from build123d import *

# Parameters (mm, degrees)
ESBO_O1_W                = 125
ESBO_O1_H                = 175
RESSALTO_EXTRUS_O1_DEPTH = 5
ESBO_O2_W                = 2.5
ESBO_O2_H                = 49
RESSALTO_EXTRUS_O2_DEPTH = 5.4
FILETE1_R                = 2
ESBO_O3_R                = 1.35
CORTE_EXTRUS_O2_DEPTH    = 140.879984272
CORTE_EXTRUS_O3_DEPTH    = 108.664571703


with BuildPart() as part:
    # Esboço1 → Ressalto-extrusão1 (new body)
    with BuildSketch(Plane.XY):
        Rectangle(ESBO_O1_W, ESBO_O1_H)
    extrude(amount=RESSALTO_EXTRUS_O1_DEPTH)

    # Esboço2 → Ressalto-extrusão2 (add)
    with BuildSketch(Plane(origin=(0, 0, 0), x_dir=(-1, 0, 0), z_dir=(0, 0, -1))):
        with Locations((7.75, 0)):
            Rectangle(ESBO_O2_W, ESBO_O2_H)
        with Locations((45.25, 0)):
            Rectangle(ESBO_O2_W, ESBO_O2_H)
    extrude(amount=RESSALTO_EXTRUS_O2_DEPTH)

    # Filete1
    filete1_edges = [part.edges().sort_by_distance(p)[0] for p in [
        (-7.75, 24.5, -5.4),
        (-7.75, -24.5, -5.4),
        (-45.25, 24.5, -5.4),
        (-45.25, -24.5, -5.4),
    ]]
    fillet(filete1_edges, radius=FILETE1_R)

    # Esboço3 → Corte-extrusão2 (cut, through all)
    with BuildSketch(Plane.ZY.offset(46.5)):
        with Locations(Location((-2.7, -21.9, 0), (0, 0, 270))):
            Circle(ESBO_O3_R)
        with Locations(Location((-2.7, 21.9, 0), (0, 0, 270))):
            Circle(ESBO_O3_R)
        with Locations(Location((-2.7, 0, 0), (0, 0, 270))):
            Circle(ESBO_O3_R)
    extrude(amount=-CORTE_EXTRUS_O2_DEPTH, mode=Mode.SUBTRACT)

    # Esboço4 → Corte-extrusão3 (cut, through all)
    with BuildSketch(Plane(origin=(0, 0, 0), x_dir=(-1, 0, 0), z_dir=(0, 0, -1))):
        Polygon((62.5, -87.5), (62.5, -69.5), (-37.5, -69.5), (-37.5, 69.5), (62.5, 69.5), (62.5, 87.5), (-62.5, 87.5), (-62.5, -87.5), align=None)
    extrude(amount=-CORTE_EXTRUS_O3_DEPTH, mode=Mode.SUBTRACT)


solid = part.part
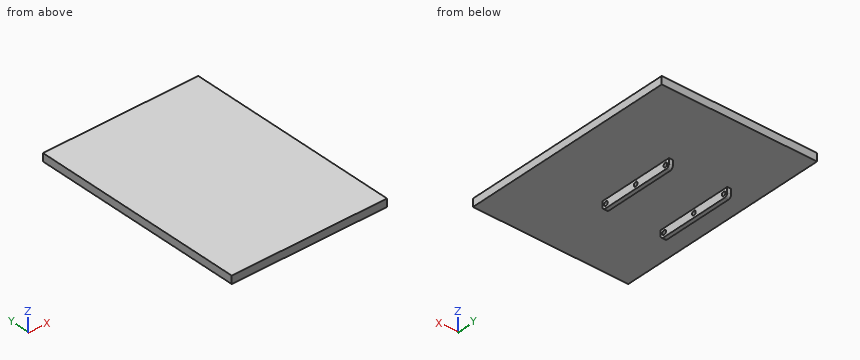
Can you work these out from the model? Positions are in its coordinate system, mm. Coordinates: 2 decimals unless noted, no trailing zeros. Loops run counter-clockwise (first coordinate to the right, second up) from the corner with the lowest first, then second, coordinate; pieces in that order, holes last. Notation, with made-up numbers: (-12, 70.25) - (35, 70.25) arc R31 ccw to (35, 105.25) - close; hole circle Ø7 at (-3, 89). An arc over 180 degrees is marked (long way). Answer as a JSON object with one key per item and string values. Group by question number.
Item 1: If we section it at C-C (y = -55.5): List the corners of the cut face in (x, z) for me, plus the area to 3 significant figures.
Item 2: If we section it at B-B (x = 21.5): List the corners of the cut face in (y, z) for me, plus the area to 3 significant figures.
Item 3: If we section it at A-A (y = 14.5): List the corners of the cut face in (x, z) for me, plus the area to 3 significant figures.
Item 4: For pin 1 (3 mm diameter, centred on x = -45.5, z = -3.5, fed in from -Y); pin 2 (1.6 mm diameter, centred on y = -3.5, z = -2, fed in from -X); pin 3 (2 mm diameter, centred on y = 21.9, z = -2.7, fed in from -X) (3 decimals); pin 4 (3 mm diameter, centred on y = -21.9, z = -2.7, fed in from +X), each with a flat end and sliding along its axis, tell me the tip position at first contact or that it passes through.
Item 5: If I drill on L1, parallel to Z at x = -44.7, y = -21.9; L2, parallel to X at y = 5, z = -4.25; L3, parallel to Z at x = -3, y = -9.5, over which ranges is the centre line in solid material (lowest first)? Write a range as from..to.
Returned:
{
 "1": {"outline": "(-62.5, 0) - (37.5, 0) - (37.5, 5) - (-62.5, 5) - close", "area": "500 mm²"},
 "2": {"outline": "(-69.5, 0) - (69.5, 0) - (69.5, 5) - (-69.5, 5) - close", "area": "695 mm²"},
 "3": {"outline": "(-62.5, 0) - (-46.5, 0) - (-46.5, -5.4) - (-44, -5.4) - (-44, 0) - (-9, 0) - (-9, -5.4) - (-6.5, -5.4) - (-6.5, 0) - (37.5, 0) - (37.5, 5) - (-62.5, 5) - close", "area": "527 mm²"},
 "4": {"pin 1": "stops at y = -24.5", "pin 2": "stops at x = -46.5", "pin 3": "passes through", "pin 4": "stops at x = -6.5"},
 "5": {"L1": "z = -5.4..-4.05, -1.35..5", "L2": "x = -46.5..-44, -9..-6.5", "L3": "z = 0..5"}
}
